Check sheet for the modelled part. Datum: model origin and axes. Units: mm. Face numbers are marked on the shaded views. A direction names the side the tool comes from. Give positions to 0.01 mm unless a question says otherwise; leave off trailing zeros. Write each loop counter-clockwise with the first axis right and the second up, starting at its lowest first coordinate (ties: lowest second). Pieces come first, ordered by that corner, then holes. Notation, with made-up numbers: (32.25, 20.5) -> (82.25, 20.5) arc R25 ccw to (82.25, 36.5) -> close; hole circle Ø10 at (-6.5, 41). An arc over 180 degrees is marked (long way). Return JSON: item names as keys, results as strings.
from build123d import *

# Parameters (mm, degrees)
F0_W     = 7.5
F0_H     = 15
F1_DEPTH = 11
F2_W     = 7
F2_H     = 3.5
F3_DEPTH = 20
F4_W     = 9
F4_H     = 5
F5_DEPTH = 4
F6_W     = 6.512857
F6_H     = 3
F7_DEPTH = 25
F8_W     = 6.512857
F8_H     = 7
F9_DEPTH = 25


with BuildPart() as f1:
    # F0 (on Right) → F1 (new body)
    with BuildSketch(Plane.YZ):
        Rectangle(F0_W, F0_H)
    extrude(amount=F1_DEPTH)

    # F2 (on face) → F3 (cut)
    with BuildSketch(Plane.XY.offset(7.5)):
        with Locations((5.5, 0)):
            Rectangle(F2_W, F2_H)
    extrude(amount=-F3_DEPTH, mode=Mode.SUBTRACT)

    # F4 (on face) → F5 (cut)
    with BuildSketch(Plane(origin=(0, 0, -7.5), x_dir=(1, 0, 0), z_dir=(0, 0, -1))):
        with Locations((5.5, 0)):
            Rectangle(F4_W, F4_H)
    extrude(amount=-F5_DEPTH, mode=Mode.SUBTRACT)

    # F6 (on face) → F7 (cut)
    with BuildSketch(Plane.XZ.offset(3.75)):
        with Locations((5.480695, 6)):
            Rectangle(F6_W, F6_H)
    extrude(amount=-F7_DEPTH, mode=Mode.SUBTRACT)

    # F8 (on Front) → F9 (cut)
    with BuildSketch(Plane.XZ):
        with Locations((5.480695, 1)):
            Rectangle(F8_W, F8_H)
    extrude(amount=-F9_DEPTH, mode=Mode.SUBTRACT)


solid = f1.part
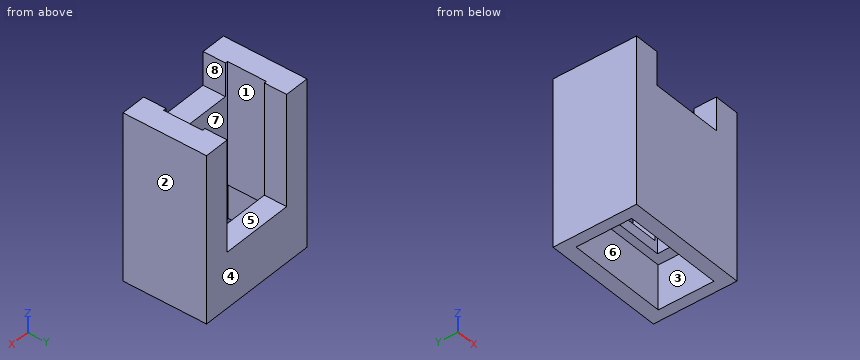
(1) Release check for a two-part mould opening along X. For the marked faces 1, 2, 3 and 4 record: pulls with the +X half, pulls with the -X half, needs draft (parallel to the pull), parting line crosses it, or undercut.
Reply:
{"face 1": "undercut", "face 2": "pulls with the +X half", "face 3": "undercut", "face 4": "needs draft"}
(2) Cross-section at A-A on y = 1.25. Enter the section's corners in (x, z), then the cut area to 3 significant figures.
Reply:
{"outline": "(0, -7.5) -> (1, -7.5) -> (1, -3.5) -> (2, -3.5) -> (2, 7.5) -> (0, 7.5) -> close; (9, -3.5) -> (10, -3.5) -> (10, -7.5) -> (11, -7.5) -> (11, 7.5) -> (9, 7.5) -> close", "area": "52.0 mm^2"}
(3) Cross-section at D-D on z = -4.5. Enter the section's corners in (x, y), then the cut area to 3 significant figures.
Reply:
{"outline": "(0, -3.75) -> (11, -3.75) -> (11, 3.75) -> (0, 3.75) -> close; hole (1, -2.5) -> (10, -2.5) -> (10, 2.5) -> (1, 2.5) -> close", "area": "37.5 mm^2"}
(4) Depth check by flat-ended pin: pin 1 Ø1.6 at (x, y) = (5.5, -3) entering from +Z; pin 2 Ø2 at (x, y) = (5.5, 2.5) entering from +Z. Enter the tip coordinate at first touch or a pass-through.
Reply:
{"pin 1": "z = 4.5", "pin 2": "z = -2.5"}
(5) Cross-section at C-C on z = 6.5. Enter the section's corners in (x, y), then the cut area to 3 significant figures.
Reply:
{"outline": "(0, -3.75) -> (2.22, -3.75) -> (2.22, -1.75) -> (2, -1.75) -> (2, 1.75) -> (2.22, 1.75) -> (2.22, 3.75) -> (0, 3.75) -> close; (8.74, -3.75) -> (11, -3.75) -> (11, 3.75) -> (8.74, 3.75) -> (8.74, 1.75) -> (9, 1.75) -> (9, -1.75) -> (8.74, -1.75) -> close", "area": "31.9 mm^2"}
(6) Set-up check for the marked faces 5, 6, 7 and 8: record each of +Z, -Z, +X, -X, +Y, -Y from which the full face is reachable in a straight line by a thin tool's end or side.
Reply:
{"face 5": "+Z, +Y", "face 6": "-Z", "face 7": "+Z, -Z", "face 8": "+Z, +Y, -Y"}
(7) Cross-section at B-B on x = 6.75. Enter the section's corners in (y, z).
Reply:
{"outline": "(-3.75, -7.5) -> (-2.5, -7.5) -> (-2.5, -3.5) -> (-1.75, -3.5) -> (-1.75, 4.5) -> (-3.75, 4.5) -> close; (1.75, -3.5) -> (2.5, -3.5) -> (2.5, -7.5) -> (3.75, -7.5) -> (3.75, -2.5) -> (1.75, -2.5) -> close"}
(8) Thickness scan on L1, parallel to X at y = -1, z = 6.25; L2, parallel to X at y = 2, z = -4; L3, parallel to Y at x = 3.5, z = -5.5. Record the ranges inside material, lowest first.
Reply:
{"L1": "0 to 2, 9 to 11", "L2": "0 to 1, 10 to 11", "L3": "-3.75 to -2.5, 2.5 to 3.75"}
